The figure shows three views and two pictorial views of one solid part (mm, origin at its lowest corner). Answer the questions. A direction names the side the tool comes from. Coordinates: 2 decimals unless noted, no trailing zeros. Loops run counter-clockwise (first coordinate to the right, second up) from the corner with the lowest first, then second, coordinate; pieces in that order, holes last.
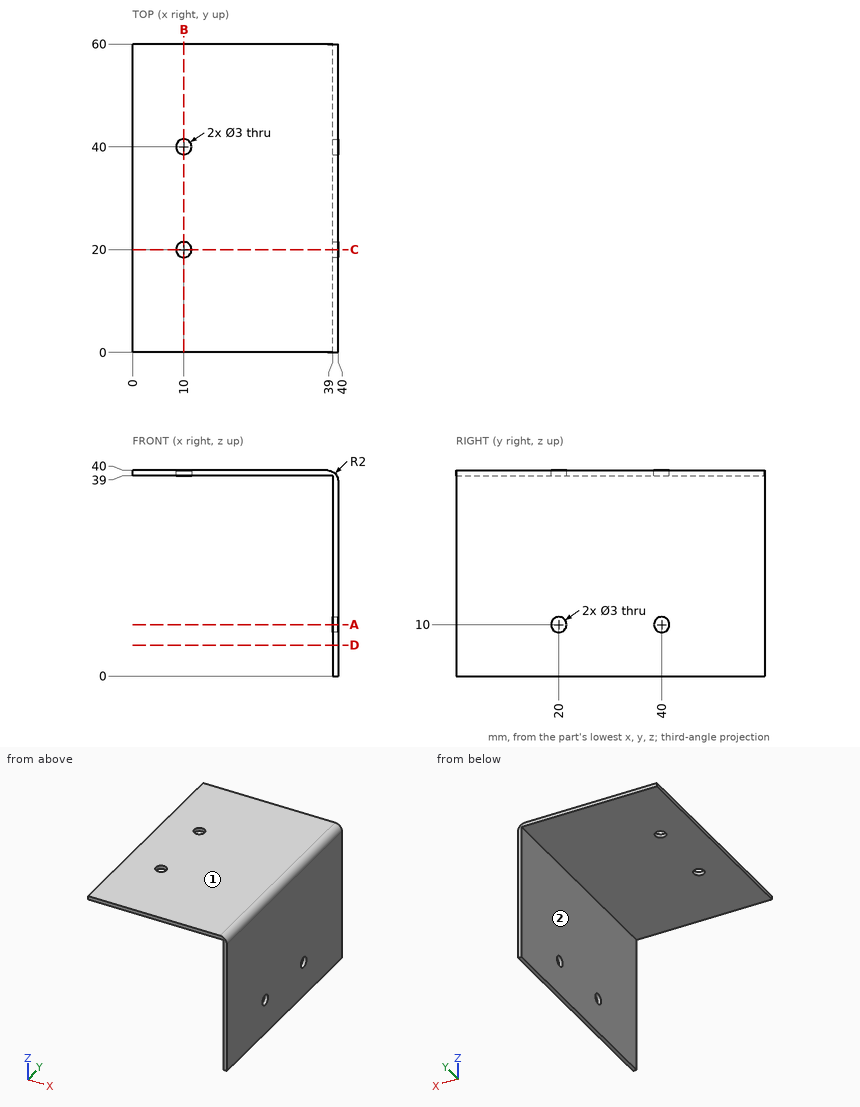
Q1. Straight lines are drawn through the part: probe 1 along Y at (x, z) = (39.55, 10); probe 2 along Z at (x, y) = (23.5, 16). For each, find the intervals that lie inside material, in ascending order.
Findings below:
probe 1: y = 0 to 18.5, 21.5 to 38.5, 41.5 to 60
probe 2: z = 39 to 40
Q2. Which of the six approach directions +Z, -Z, +X, -X, +Y, -Y give full straight-line access (tool end or side, diameter ignored) to the marked faces 1 and 2?
Findings below:
face 1: +Z, +X, -X, +Y, -Y
face 2: -Z, -X, +Y, -Y
Q3. A cutting plane is placed at B-B (x = 10). Give the vertices of the cut face in (y, z).
Findings below:
outline: (0, 39) - (18.5, 39) - (18.5, 40) - (0, 40) - close; (21.5, 39) - (38.5, 39) - (38.5, 40) - (21.5, 40) - close; (41.5, 39) - (60, 39) - (60, 40) - (41.5, 40) - close
Q4. Flat-ended cylindrical pins translate along their axes: pin 1 Ø4 at (x, y) = (5, 15) entering from -Z; pin 2 Ø2.5 at (x, y) = (10, 40) entering from +Z; pin 3 Ø5 at (y, z) = (46, 22.5) entering from -X. Find the tip coordinate at first contact, or state that the pin passes through.
Findings below:
pin 1: stops at z = 39
pin 2: passes through
pin 3: stops at x = 39
Q5. A cutting plane is placed at D-D (z = 6). Give the vertices of the cut face in (x, y), then the cut area to 3 significant figures.
Findings below:
outline: (39, 0) - (40, 0) - (40, 60) - (39, 60) - close
area: 60.0 mm2
Q6. A cutting plane is placed at A-A (z = 10). Give the vertices of the cut face in (x, y), then the cut area to 3 significant figures.
Findings below:
outline: (39, 0) - (40, 0) - (40, 18.5) - (39, 18.5) - close; (39, 21.5) - (40, 21.5) - (40, 38.5) - (39, 38.5) - close; (39, 41.5) - (40, 41.5) - (40, 60) - (39, 60) - close
area: 54.0 mm2
Q7. A cutting plane is placed at C-C (y = 20). Give the vertices of the cut face in (x, z), then the cut area to 3 significant figures.
Findings below:
outline: (0, 39) - (8.5, 39) - (8.5, 40) - (0, 40) - close; (11.5, 39) - (39, 39) - (39, 11.5) - (40, 11.5) - (40, 38) arc R2 ccw to (38, 40) - (11.5, 40) - close; (39, 0) - (40, 0) - (40, 8.5) - (39, 8.5) - close
area: 72.1 mm2
